Here's how the part is built. I have some questions about the finished solid (model axes, mm). A direction names the side the tool comes from. Round coordinates to 2 decimals unless told otherwise and drop trailing zeros. Loops run counter-clockwise (first coordinate to the right, second up) from the corner with the lowest first, then second, coordinate; pieces in that order, holes last. Notation, with made-up numbers: M 80,-32 L 108,-32 A17 ccw 108,-28 Z; hole C 88,81 d4. An arc over 180 degrees is marked long. Use a Markdown table: item, result.
from build123d import *

# Parameters (mm, degrees)
SKETCH_R           = 18
PAD_DEPTH          = 3
SKETCH001_R        = 15
PAD001_DEPTH       = 108
SKETCH002_R        = 9.5
PAD002_DEPTH       = 2.5
SKETCH003_R        = 13
PAD003_DEPTH       = 5.5
PAD004_DEPTH       = 1.5
POLARPATTERN_COUNT = 6
SKETCH009_W        = 8
SKETCH009_H        = 10
POCKET_DEPTH       = 118
SKETCH010_R        = 4.15
POCKET001_DEPTH    = 10
SKETCH011_R        = 4.15
POCKET002_DEPTH    = 10
SKETCH012_W        = 10
SKETCH012_H        = 32.3
POCKET003_DEPTH    = 14


with BuildPart() as part:
    # Sketch → Pad (new body)
    with BuildSketch(Plane.XY):
        Circle(SKETCH_R)
    extrude(amount=PAD_DEPTH)

    # Sketch001 (on Face3 of Pad) → Pad001 (join)
    with BuildSketch(Plane.XY.offset(3)):
        Circle(SKETCH001_R)
    extrude(amount=PAD001_DEPTH)

    # Sketch002 (on Face2 of Pad001) → Pad002 (join)
    with BuildSketch(Plane(origin=(0, 0, 0), x_dir=(1, 0, 0), z_dir=(0, 0, -1))):
        Circle(SKETCH002_R)
    extrude(amount=PAD002_DEPTH)

    # Sketch003 (on Face7 of Pad002) → Pad003 (join)
    with BuildSketch(Plane.XY.offset(111)):
        Circle(SKETCH003_R)
    extrude(amount=PAD003_DEPTH)

    # Sketch008 (on Face3 of Pad003) → Pad004 (join)
    with BuildSketch(Plane.XY.offset(3)):
        Polygon((-1.11579, 17.121659), (-0.012041, 17.758909), (1.091708, 17.121659), (1.091708, 15.84716), (-0.012041, 15.209911), (-1.11579, 15.84716), align=None)
    pad004 = extrude(amount=PAD004_DEPTH)

    # PolarPattern: Pad004 ×6 about axis
    polarpattern_axis = Axis((0, 0, 3), (0, 0, 1))
    for i in range(1, POLARPATTERN_COUNT):
        add(pad004.rotate(polarpattern_axis, i * 360 / POLARPATTERN_COUNT))

    # Sketch009 (on Face2 of PolarPattern) → Pocket (cut)
    with BuildSketch(Plane(origin=(0, 0, 0), x_dir=(1, 0, 0), z_dir=(0, 0, -1))):
        with Locations((-14, 0)):
            Rectangle(SKETCH009_W, SKETCH009_H)
    extrude(amount=-POCKET_DEPTH, mode=Mode.SUBTRACT)

    # Sketch010 (on DatumPlane) → Pocket001 (cut)
    with BuildSketch(Plane.XZ.offset(15)):
        with Locations((0, 87)):
            Circle(SKETCH010_R)
    extrude(amount=-POCKET001_DEPTH, mode=Mode.SUBTRACT)

    # Sketch011 (on DatumPlane) → Pocket002 (cut)
    with BuildSketch(Plane.XZ.offset(15)):
        with Locations((0, 63)):
            Circle(SKETCH011_R)
    extrude(amount=-POCKET002_DEPTH, mode=Mode.SUBTRACT)

    # Sketch012 (on Face7 of Pocket002) → Pocket003 (cut)
    with BuildSketch(Plane(origin=(-10, 0, 0), x_dir=(0, -1, 0), z_dir=(-1, 0, 0))):
        with Locations((0, 75)):
            Rectangle(SKETCH012_W, SKETCH012_H)
    extrude(amount=-POCKET003_DEPTH, mode=Mode.SUBTRACT)


solid = part.part
1. We'd pull the mould along X, two halves only. Please class faces 4 (the face through (13, 0, 114)), 5 (the face through (14, 8, 4.5)), 6 (the face through (-4.146, -10.071, 87.182)): +X half, -X half, draft (parallel to the pull), parting line (faces both ways), or undercut.
Answer sheet:
| item | result |
|---|---|
| face 4 | parting line |
| face 5 | draft |
| face 6 | undercut |
2. For pin 1 Ø2 at (y, z) = (-14, 58) entering from +X; pin 2 Ø10 at (y, z) = (8, 83) entering from +X; pin 3 Ø0.6 at (y, z) = (8.5, 3.5) entering from -X; pin 4 Ø12 at (x, y) = (-12.5, 0) entering from +Z, each with a flat end and sliding along its axis, tell me the tip position at first contact or that it passes through.
Answer sheet:
| item | result |
|---|---|
| pin 1 | x = 7.48 |
| pin 2 | x = 14.7 |
| pin 3 | x = -15.39 |
| pin 4 | z = 116.5 |
3. Imagine slicing it at C-C, the plane y = 0. Write out the boundary of the cut face in (x, z), then the cut area to 3 significant figures.
Answer sheet:
| item | result |
|---|---|
| outline | M -10,0 L -9.5,0 L -9.5,-2.5 L 9.5,-2.5 L 9.5,0 L 18,0 L 18,3 L 15,3 L 15,111 L 13,111 L 13,116.5 L -10,116.5 L -10,91.15 L 4,91.15 L 4,58.85 L -10,58.85 Z |
| area | 2,510 mm2 |
4. Imagine slicing it at B-B, the plane x = -5.5. Write out the boundary of the cut face in (y, z).
Answer sheet:
| item | result |
|---|---|
| outline | M -17.14,0 L -7.75,0 L -7.75,-2.5 L 7.75,-2.5 L 7.75,0 L 17.14,0 L 17.14,3 L 13.96,3 L 13.96,111 L 11.78,111 L 11.78,116.5 L -11.78,116.5 L -11.78,111 L -13.96,111 L -13.96,3 L -17.14,3 Z; hole M -5,58.85 L 5,58.85 L 5,91.15 L -5,91.15 Z |
5. Which directions (+Z, -Z, +X, -X, +Y, -Y) give clear straight access to the entire face, cutting with the end or side of a thin tool? Please do faces 1 (the face through (0, -17, 4.5)), 2 (the face through (8, -8, 0)), 3 (the face through (13.3, 0.1, 111)).
Answer sheet:
| item | result |
|---|---|
| face 1 | +Z, +X, -X, -Y |
| face 2 | -Z |
| face 3 | +Z |
6. I need wall thicknesses on probe 1 along Z at (x, y) = (0, -8); probe 2 along Z at (x, y) = (0, -11.25); probe 3 along Z at (x, y) = (3, 2). Which ranges of each line are inside material? Lowest first, please. Write a range as from..to.
Answer sheet:
| item | result |
|---|---|
| probe 1 | -2.5..58.85, 67.15..82.85, 91.15..116.5 |
| probe 2 | 0..58.85, 67.15..82.85, 91.15..116.5 |
| probe 3 | -2.5..58.85, 91.15..116.5 |
7. Imagine slicing it at A-A, the plane z = 63. Write out the boundary of the cut face in (x, y), then the cut area to 3 significant figures.
Answer sheet:
| item | result |
|---|---|
| outline | M -14.14,-5 A15 ccw -4.15,-14.41 L -4.15,-5 Z; M -14.14,5 L 4,5 L 4,-5 L 4.15,-5 L 4.15,-14.41 A15 ccw long Z |
| area | 438 mm2 |
